Geometry: final body of the model. Coordinates: model frame, mm. A direction names the side the tool comes from. Coordinates: 2 decimals unless noted, no trailing zeros. Write each loop counter-clockwise with the first axis right and the second up, starting at its lowest first coordinate (ties: lowest second). Pieces come first, ordered by that corner, then holes. Notation, with made-up numbers: (-24.5, 86.25) - (4.5, 86.25) arc R17 cw to (4.5, 99.25) - close; hole circle Ø1 at (40, 46). An arc over 180 degrees is marked (long way). Put each result on its own line as item: value.
Autodesk Inventor part; units mm, degrees
ref_plane "作業平面1" through (-5, 20.1603, 5.5) normal (0, -1, 0) x (1, 0, 0)
ref_plane "YZ Plane" through (0, 0, 0) normal (1, 0, 0) x (0, 1, 0)
ref_plane "XZ Plane" through (0, 0, 0) normal (0, 1, 0) x (-1, 0, 0)
sketch "スケッチ1" plane through (0, 0, 0) normal (0, 0, 1) x (1, 0, 0)
  line L0 (-17.5, 0) -> (17.5, 0)
  line L1 (17.5, 0) -> (17.5, 59.5)
  line L2 (17.5, 59.5) -> (-17.5, 59.5)
  line L3 (-17.5, 59.5) -> (-17.5, 0)
  line L4 (-12.5, 59.5) -> (12.5, 59.5)
  line L5 (12.5, 59.5) -> (12.5, 65)
  line L6 (12.5, 65) -> (-12.5, 65)
  line L7 (-12.5, 65) -> (-12.5, 59.5)
  point P0 (0, 0)
  point P1 (0, 0)
  point P2 (0, 59.5)
  dimension "d0" = 59.5
  dimension "d1" = 35
  dimension "d2" = 25
  dimension "d3" = 5.5
extrude "押し出し1" add sketch "スケッチ1" along normal blind 5.5
sketch "スケッチ2" plane through (0, 0, 5.5) normal (0, 0, 1) x (1, 0, 0)
  line L0 (-13, 10) -> (-3, 10)
  line L1 (-13, 10) -> (-8, 18.6603)
  line L2 (-8, 18.6603) -> (-3, 10)
  line L3 (0, 10) -> (5, 18.6603)
  line L4 (5, 18.6603) -> (-5, 18.6603)
  line L5 (-5, 18.6603) -> (0, 10)
  line L6 (3, 10) -> (13, 10)
  line L7 (13, 10) -> (8, 18.6603)
  line L8 (8, 18.6603) -> (3, 10)
  line L9 (0, -13) -> (0, 78)
  line L10 (-17.5, 0) -> (17.5, 0)
  line L11 (-11, 18.6603) -> (-16, 10)
  line L12 (-16, 10) -> (-16, 18.6603)
  line L13 (-16, 18.6603) -> (-11, 18.6603)
  line L14 (-13.5, 18.6603) -> (-13.5, 10)
  point P0 (0, 0)
  point P1 (0, 18.6603)
  point P2 (-13.5, 14.3301)
  dimension "d6" = 10
  dimension "d7" = 3
  dimension "d8" = 10
  dimension "d9" = 3
extrude "押し出し2" cut sketch "スケッチ2" against normal through all contours L1 L2 L0 | L5 L4 L9 | L11 L14 L13
ref_plane "作業平面1" through (-5, 20.1603, 5.5) normal (0, -1, 0) x (1, 0, 0)
mirror "ミラー1" about plane through (-5, 20.1603, 5.5) normal (0, -1, 0) of "押し出し2"
pattern_linear "矩形状パターン1" count 2 spacing 23.3 along (0, 1, 0) of "押し出し2", "ミラー1"
mirror "ミラー2" about plane through (0, 0, 0) normal (1, 0, 0) of "押し出し2", "ミラー1", "矩形状パターン1"
equation "\"d9\" = d7"
properties part number "motor_setter_spacer"
1. Mould query, pull axis Y, two halves, no side actions, for faces 1 (the flat face through (2.465, 14.27, 2.788)), 2 (the flat face through (0, 33, 0)), 3 (the flat face through (12.233, 47.095, 2.788)). Classes: +Y half, -Y half, draft (parallel to the pull), parting line (faces both ways), or undercut.
Answer below:
face 1: undercut
face 2: draft
face 3: undercut
2. Section query B-B (x = 9). Return loops of the section in (y, z).
Answer below:
outline: (0, 0) - (10, 0) - (10, 5.5) - (0, 5.5) - close; (16.93, 0) - (23.39, 0) - (23.39, 5.5) - (16.93, 5.5) - close; (30.32, 0) - (33.3, 0) - (33.3, 5.5) - (30.32, 5.5) - close; (40.23, 0) - (46.69, 0) - (46.69, 5.5) - (40.23, 5.5) - close; (53.62, 0) - (65, 0) - (65, 5.5) - (53.62, 5.5) - close
3. Ray query, probe 1 along Y at (x, z) = (-10.5, 4.5); probe 2 along X at (y, z) = (52, 5.1); probe 3 along Y at (x, z) = (-6.5, 5.15). Return the intervals inside material, ascending. Write a range as from..to.
Answer below:
probe 1: y = 0..10, 14.33..25.99, 30.32..33.3, 37.63..49.29, 53.62..65
probe 2: x = -17.5..-12.06, -3.94..-0.94, 0.94..3.94, 12.06..17.5
probe 3: y = 0..10, 16.06..24.26, 30.32..33.3, 39.36..47.56, 53.62..65
4. Section query D-D (z = 2.9). Count the separate pieces of the cut face and the enclosed holes in it, then the cut area to 3 significant figures.
Answer below:
separate pieces: 1
enclosed holes: 20
area: 1,660 mm²
5. Section query C-C (y = 28). Return loops of the section in (x, z).
Answer below:
outline: (-17.5, 0) - (-11.66, 0) - (-11.66, 5.5) - (-17.5, 5.5) - close; (-4.34, 0) - (-1.34, 0) - (-1.34, 5.5) - (-4.34, 5.5) - close; (1.34, 0) - (4.34, 0) - (4.34, 5.5) - (1.34, 5.5) - close; (11.66, 0) - (17.5, 0) - (17.5, 5.5) - (11.66, 5.5) - close
6. Pin query (flat end, axial travel): pin 1 Ø2.5 at (x, z) = (-16, 4) entering from +Y. Return the tip coordinate at first contact, or that it passes through.
Answer below:
pin 1: stops at y = 59.5
7. Set-up query: faces 4 (the flat face through (5.465, 14.27, 2.788)), 5 (the flat face through (0, 33, 5.5)). Return all of +Z, -Z, +X, -X, +Y, -Y with unobstructed straight access to the full face (end or side cutting, diameter ignored); none if empty.
Answer below:
face 4: +Z, -Z
face 5: +Z, +X, -X, +Y, -Y
8. Section query A-A (y = 17). Return loops of the section in (x, z).
Answer below:
outline: (-17.5, 0) - (-13.5, 0) - (-13.5, 5.5) - (-17.5, 5.5) - close; (-11.96, 0) - (-8.96, 0) - (-8.96, 5.5) - (-11.96, 5.5) - close; (-7.04, 0) - (-4.04, 0) - (-4.04, 5.5) - (-7.04, 5.5) - close; (4.04, 0) - (7.04, 0) - (7.04, 5.5) - (4.04, 5.5) - close; (8.96, 0) - (11.96, 0) - (11.96, 5.5) - (8.96, 5.5) - close; (13.5, 0) - (17.5, 0) - (17.5, 5.5) - (13.5, 5.5) - close
